Answer from the drawing. Dimensions are ordinates in mm from the lowest x, y and z of the part. A direction names the side the tool comes from. Round coordinates to 2 decimals unless told otherwise and drop trailing zeros. Write each loop counter-clockwise with the first axis right and the second up, starting at its lowest first coordinate (ties: lowest second). Pieces come first, ordered by that corner, then holes.
1. Find section C-C (y = 0.75). Write down the section's boundary in (x, z), and give its area (3 significant figures).
2. A tool of negligible diameter and unlimited length cuts with its end or side. For the marked faces 4 and 5, from which of +Z, -Z, +X, -X, +Y, -Y can it reach the whole face along a straight path? Write none if from no direction.
3. Straight lines are drawn through the part: probe 1 along Z at (x, y) = (2, 6.25); probe 2 along Y at (x, z) = (3.2, 2.45); probe 3 along X at (y, z) = (2.25, 1.1). For each, find the intervals that lie inside material, in ascending order.
4. Determine the mould class of the marked faces 1, 2 and 3 for opening direction Y: pulls with the +Y half, pulls with the -Y half, needs draft (parallel to the pull), parting line crosses it, or undercut.
5. Flat-ended cylindrical pins translate along their axes: pin 1 Ø1.5 at (x, y) = (3.5, 4.5) entering from -Z; pin 2 Ø2 at (y, z) = (1.5, 3) entering from -X. Find the tip coordinate at first contact, or state that the pin passes through.
6. Find section D-D (y = 3.5). Write down the section's boundary in (x, z), and give its area (3 significant figures).
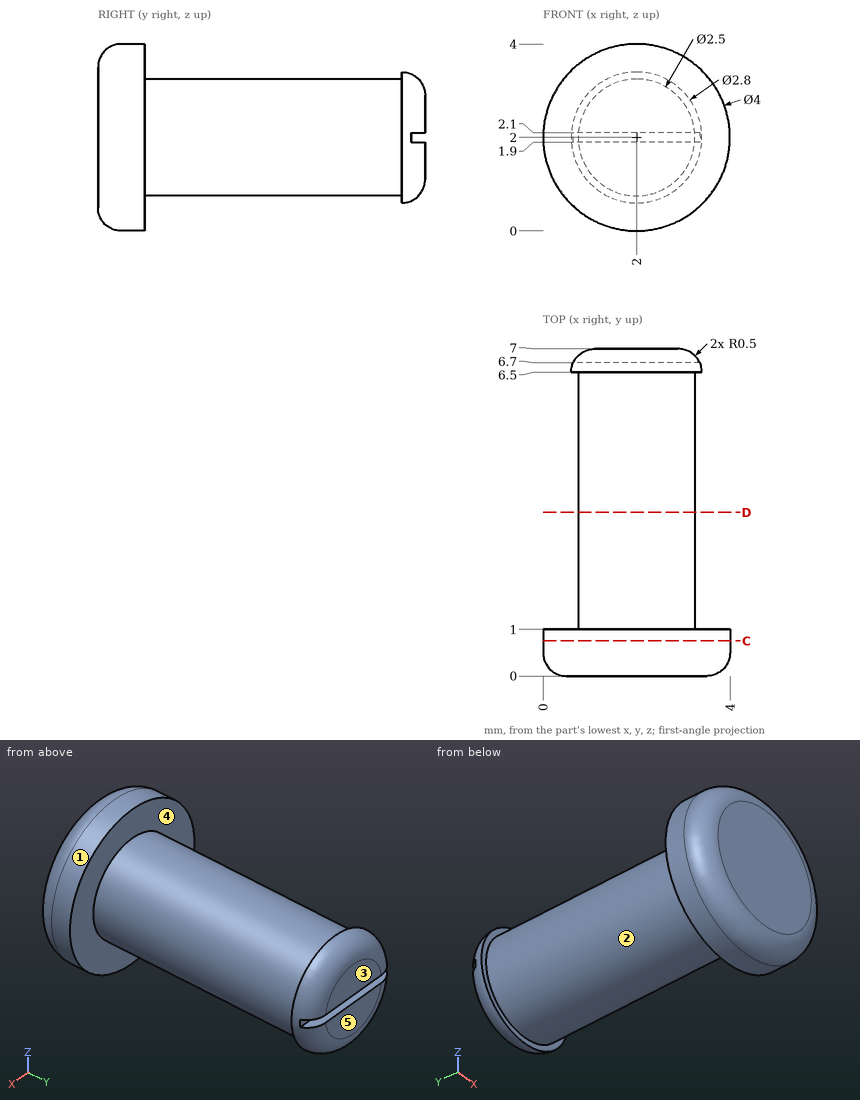
Worked answers:
1. outline: circle Ø4 at (2, 2)
1. area: 12.6 mm2
2. face 4: none
2. face 5: +Z, -Z, +X, -X, +Y
3. probe 1: z = 0.75 to 3.25
3. probe 2: y = 0 to 1, 6.5 to 6.82
3. probe 3: x = 1.13 to 2.87
4. face 1: needs draft
4. face 2: undercut
4. face 3: pulls with the +Y half
5. pin 1: stops at z = 1
5. pin 2: stops at x = 0
6. outline: circle Ø2.5 at (2, 2)
6. area: 4.91 mm2
